from build123d import *

# Parameters (mm, degrees)
F0_W     = 101.6
F0_H     = 50.8
F1_DEPTH = 1.27
F2_W     = 69.85
F2_H     = 3.175
F2_W_2   = 6.35
F2_H_2   = 45.72
F3_DEPTH = 7.62
F4_W     = 21.532409323
F4_H     = 15.0506472416
F4_W_2   = 14.7617278114
F4_H_2   = 7.62
F5_DEPTH = 12.7
F6_R     = 3.80999


# Not quite as in the source:
# - a fillet or chamfer is up to 0.001 mm smaller than in the source, because OpenCascade refuses the exact size


with BuildPart() as f1:
    # F0 (on Top) → F1 (new body)
    with BuildSketch(Plane.XY):
        Rectangle(F0_W, F0_H)
    extrude(amount=F1_DEPTH)

    # F2 (on face) → F3 (join)
    with BuildSketch(Plane.XY.offset(1.27)):
        with Locations((3.175, 21.2725)):
            Rectangle(F2_W, F2_H)
        with Locations((45.085, 0)):
            Rectangle(F2_W_2, F2_H_2)
        with Locations((3.175, -21.2725)):
            Rectangle(F2_W, F2_H)
    extrude(amount=F3_DEPTH)

    # F4 (on face) → F5 (join)
    with BuildSketch(Plane.XY.offset(1.27)):
        with Locations((-35.9846150789, 9.7787969645)):
            Rectangle(F4_W, F4_H)
        with Locations((-38.3539574899, -9.3564780889)):
            Rectangle(F4_W_2, F4_H_2)
    extrude(amount=F5_DEPTH)

    # F6 (radius 3.81 in the source; OpenCascade refuses exactly that, so slightly less here)
    f6_edges = [f1.edges().sort_by_distance(p)[0] for p in [
        (-38.353957, -13.166478, 13.97),
        (-38.353957, -5.546478, 13.97),
    ]]
    fillet(f6_edges, radius=F6_R)


solid = f1.part
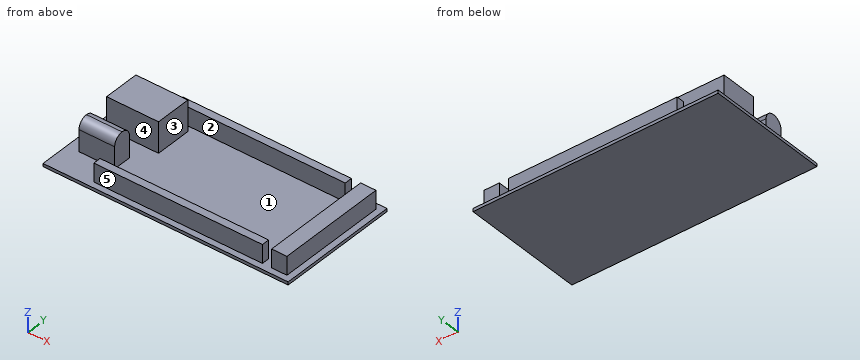
Check sheet for the modelled part. Datum: model origin and axes. Units: mm. Face numbers are marked on the shaded views. A direction names the side the tool comes from. Give positions to 0.01 mm unless a question says otherwise; leave off trailing zeros. Write each loop counter-clockwise with the first axis right and the second up, starting at its lowest first coordinate (ties: lowest second). Pieces come first, ordered by that corner, then holes. Notation, with made-up numbers: (85, 29) -> (101, 29) arc R31 ccw to (101, 53) -> close; hole circle Ø11 at (4.25, -14). An arc over 180 degrees is marked (long way). One line per item, written item: value. Start each with the question number.
Item 1: Section check D-D on x = 19.5. Record the cut outline in (y, z) (3 decimals), then the cut area to 3 significant figures.
Item 2: Section check C-C on z = 11.25. Record the cut outline in (x, y).
Item 3: Material ranges on probe 1 along Y at (x, z) = (8.5, 4.75) (3 decimals); probe 2 along X at (y, z) = (-12, 6); probe 3 along Z at (x, y) = (39, -17), recorded low to high. Write a range as from..to.
Item 4: Gauge pin test, flat ends, axial feed: pin 1 (2 mm diameter, centred on x = -3, y = 10, fed in from +Z); pin 2 (2.5 mm diameter, centred on x = 17.5, z = 3.5, fed in from -Y); pin 3 (7 mm diameter, centred on x = 46, z = 4, fed in from -Y); pin 4 (1 mm diameter, centred on y = -0.5, z = 10.5, fed in from +X). Record the tip position at first contact, or that the pin passes through.
Item 5: Tool access check on the marked faces 3, 4 and 5. Record the directions out of +Z, -Z, +X, -X, +Y, -Y that give a thin tool (end or side, any length) a straight path to the whole face; none if there is none.
Item 6: Section check A-A on z = 2.5. Record the cut outline in (x, y) (3 decimals).
Item 7: Section check B-B on y = -14.5. Record the cut outline in (x, z), then the cut area to 3 significant figures.
Item 8: Draft check along X on the marked faces 1 and 2. Enter one of: +X half, -X half, draft (parallel to the pull), parting line (faces both ways), or undercut.
Results list:
1. outline: (-25.4, 0) -> (25.4, 0) -> (25.4, 1.27) -> (22.86, 1.27) -> (22.86, 8.89) -> (19.685, 8.89) -> (19.685, 1.27) -> (-19.685, 1.27) -> (-19.685, 8.89) -> (-22.86, 8.89) -> (-22.86, 1.27) -> (-25.4, 1.27) -> close
1. area: 113 mm²
2. outline: (-46.75, 2.25) -> (-25.22, 2.25) -> (-25.22, 17.3) -> (-46.75, 17.3) -> close; (-45.73, -13.01) -> (-30.97, -13.01) -> (-30.97, -5.71) -> (-45.73, -5.71) -> close
3. probe 1: -22.86..-19.685, 19.685..22.86
3. probe 2: -45.73..-30.97, 41.91..48.26
3. probe 3: 0..1.27
4. pin 1: z = 1.27
4. pin 2: y = -22.86
4. pin 3: y = -25.4
4. pin 4: through
5. face 3: +Z
5. face 4: +Z, -X
5. face 5: +Z, +X, -X, -Y
6. outline: (-46.751, 2.253) -> (-25.218, 2.253) -> (-25.218, 17.304) -> (-46.751, 17.304) -> close; (-45.735, -13.166) -> (-30.973, -13.166) -> (-30.973, -5.546) -> (-45.735, -5.546) -> close; (-31.75, -22.86) -> (38.1, -22.86) -> (38.1, -19.685) -> (-31.75, -19.685) -> close; (-31.75, 19.685) -> (38.1, 19.685) -> (38.1, 22.86) -> (-31.75, 22.86) -> close; (41.91, -22.86) -> (48.26, -22.86) -> (48.26, 22.86) -> (41.91, 22.86) -> close
7. outline: (-50.8, 0) -> (50.8, 0) -> (50.8, 1.27) -> (48.26, 1.27) -> (48.26, 8.89) -> (41.91, 8.89) -> (41.91, 1.27) -> (-50.8, 1.27) -> close
7. area: 177 mm²
8. face 1: undercut
8. face 2: draft
